from build123d import *

# Parameters (mm, degrees)
SKETCH1_W                = 25
SKETCH1_H                = 38
SKETCH1_W_2              = 16.5
SKETCH1_H_2              = 1.4
BOSS_EXTRUDE1_DEPTH      = 2
SKETCH1_3_W              = 16.5
SKETCH1_3_H              = 1.4
BOSS_EXTRUDE2_DEPTH      = 5.5
BOSS_EXTRUDE3_DEPTH      = 3
BOSS_EXTRUDE3_DEPTH_BACK = 3
SKETCH3_W                = 6.5
SKETCH3_H                = 1.4
SKETCH3_W_2              = 10
CUT_EXTRUDE1_DEPTH       = 3.5


with BuildPart() as part:
    # Sketch1 → Boss-Extrude1 (new body)
    with BuildSketch(Plane(origin=(0, 0, 0), x_dir=(1, 0, 0), z_dir=(0, 1, 0))):
        Rectangle(SKETCH1_W, SKETCH1_H)
        with Locations((0, -17.2)):
            Rectangle(SKETCH1_W_2, SKETCH1_H_2, mode=Mode.SUBTRACT)
        with Locations((0, 17.2)):
            Rectangle(SKETCH1_W_2, SKETCH1_H_2, mode=Mode.SUBTRACT)
    extrude(amount=BOSS_EXTRUDE1_DEPTH)

    # Sketch1<3> → Boss-Extrude2 (add)
    with BuildSketch(Plane(origin=(0, 0, 0), x_dir=(1, 0, 0), z_dir=(0, 1, 0))):
        Polygon((-14, -1.5), (-12.5, -3), (-12.5, 3), (-14, 1.5), align=None)
        Polygon((12.5, 3), (12.5, -3), (14, -1.5), (14, 1.5), align=None)
        with Locations((0, 17.2)):
            Rectangle(SKETCH1_3_W, SKETCH1_3_H)
        with Locations((0, -17.2)):
            Rectangle(SKETCH1_3_W, SKETCH1_3_H)
    extrude(amount=BOSS_EXTRUDE2_DEPTH)

    # Sketch2 → Boss-Extrude3 (add, two sides: drawn at the far end of the back side and taken through both)
    with BuildSketch(Plane.XY.offset(-BOSS_EXTRUDE3_DEPTH_BACK)):
        Polygon((12.5, 5.5), (11.5, 4.5), (12.5, 4.5), align=None)
        Polygon((-11.5, 4.5), (-12.5, 4.5), (-12.5, 5.5), align=None)
    extrude(amount=BOSS_EXTRUDE3_DEPTH + BOSS_EXTRUDE3_DEPTH_BACK)

    # Sketch3 → Cut-Extrude1 (cut)
    with BuildSketch(Plane(origin=(0, 2, 0), x_dir=(1, 0, 0), z_dir=(0, 1, 0))):
        with Locations((0, -17.2)):
            Rectangle(SKETCH3_W, SKETCH3_H)
        with Locations((0, 17.2)):
            Rectangle(SKETCH3_W_2, SKETCH3_H)
    extrude(amount=CUT_EXTRUDE1_DEPTH, mode=Mode.SUBTRACT)


solid = part.part
Can you work these out from the model? Positions are in its coordinate system, mm. A direction names the side the tool comes from. Give positions to 0.01 mm unless a question says otherwise; leave off trailing zeros. Order: outer loops, then holes, each group sorted by start corner. A loop starts at its lowest first (then second) coordinate and runs counter-clockwise, first axis right, second up. Notation, with made-up numbers: M 30.25,-30.5 L 58.25,-30.5 A31 cw 58.25,7.5 Z; hole C -3.5,59 d2. An arc over 180 degrees is marked long. Use one line per item in the form item = value. Start each with the question number.
Item 1: If we section it at D-D (z = 3.5): Write out the boundary of the cut face in (x, y), then the cut area to 3 significant figures.
Item 2: If we section it at A-A (z = -2): Write out the boundary of the cut face in (x, y).
Item 3: If we section it at C-C (x = -3.75): Write out the boundary of the cut face in (y, z), then the cut area to 3 significant figures.
Item 4: Will these pins go through, and if not, where does the flat tip stop? pin 1 Ø1.5 at (x, y) = (-3, 4.5) entering from -Z; pin 2 Ø1.5 at (y, z) = (3, 17.5) entering from +X; pin 3 Ø12.5 at (x, z) = (1.5, 5.5) entering from +Y; pin 4 Ø1.1 at (x, z) = (-12, -0.5) entering from -Y.
Item 5: For faces 1 (the flat face through (8.25, 4, -17)), 2 (the flat face through (-7, 4, -17.9)), 3 (the flat face through (6, 4, 17.9)), 4 (the flat face through (12, 5, 0)), which set-ups out of +Z, -Z, +X, -X, +Y, -Y let a thin tool reach every point of the face, with its end or its side?
Item 6: If we section it at B-B (x = 7): Write out the boundary of the cut face in (y, z).
Item 7: We'd pull the mould along Y, two halves only. Please class faces 5 (the flat face through (6, 5.5, 17)), 6 (the flat face through (0, 0, 0)), 7 (the flat face through (12.5, 3, 0)), 8 (the flat face through (12.2, 4.8, -3)): +Y half, -Y half, draft (parallel to the pull), parting line (faces both ways), or undercut.
Item 8: If I drill on line 1 along Z through (x, y) = (6.75, 3.1); line 2 along X through (y, z) = (1.95, 4.5); line 3 along Y through (x, z) = (1.5, -16), over which ranges is the centre line in solid material (lowest first)?
Outcome:
q1.outline = M -12.5,0 L 12.5,0 L 12.5,2 L -12.5,2 Z
q1.area = 50.0 mm2
q2.outline = M -13.5,0 L 13.5,0 L 13.5,5.5 L 12.5,5.5 L 11.5,4.5 L 12.5,4.5 L 12.5,2 L -12.5,2 L -12.5,4.5 L -11.5,4.5 L -12.5,5.5 L -13.5,5.5 Z
q3.outline = M 0,-19 L 2,-19 L 2,16.5 L 5.5,16.5 L 5.5,17.9 L 2,17.9 L 2,19 L 0,19 Z
q3.area = 80.9 mm2
q4.pin_1 = 16.5
q4.pin_2 = 8.25
q4.pin_3 = 2
q4.pin_4 = 0
q5.face_1 = +Z, -Z, +X, +Y
q5.face_2 = -Z, +X, -X, +Y
q5.face_3 = +Z, +X, -X, +Y
q5.face_4 = +Z, -Z, +Y
q6.outline = M 0,-19 L 2,-19 L 2,-17.9 L 5.5,-17.9 L 5.5,-16.5 L 2,-16.5 L 2,16.5 L 5.5,16.5 L 5.5,17.9 L 2,17.9 L 2,19 L 0,19 Z
q7.face_5 = +Y half
q7.face_6 = -Y half
q7.face_7 = undercut
q7.face_8 = draft
q8.line_1 = -17.9 to -16.5, 16.5 to 17.9
q8.line_2 = -12.5 to 12.5
q8.line_3 = 0 to 2
